```python
from build123d import *

# Parameters (mm, degrees)
PAD008_DEPTH    = 50
SKETCH046_R     = 2.4
SKETCH046_R_2   = 2
POCKET024_DEPTH = 30
SKETCH047_W     = 30
SKETCH047_H     = 35
POCKET025_DEPTH = 30
POCKET026_DEPTH = 5
FILLET014_R     = 4
FILLET015_R     = 1
FILLET016_R     = 1


with BuildPart() as part:
    # Sketch045 → Pad008 (new body)
    with BuildSketch(Plane.XZ):
        with BuildLine():
            Line((0, 47), (0, -18))
            ThreePointArc((0, -18), (0.585786, -19.414214), (2, -20))
            Line((2, -20), (23, -20))
            Line((23, -20), (23, -17.9))
            Line((17, -17.9), (23, -17.9))
            Line((17, -4.9), (17, -17.9))
            Line((17, -4.9), (23, -4.9))
            Line((23, -4.9), (23, -2))
            Line((23, -2), (9, -2))
            ThreePointArc((4, 3), (5.464466, -0.535534), (9, -2))
            Line((4, 3), (4, 47))
            Line((4, 47), (0, 47))
        make_face()
    extrude(amount=-PAD008_DEPTH)

    # Sketch046 → Pocket024 (cut)
    with BuildSketch(Plane.YZ):
        with Locations((10, -11.4)):
            Circle(SKETCH046_R)
        with Locations((10, 25)):
            Circle(SKETCH046_R_2)
        with Locations((40, 25)):
            Circle(SKETCH046_R_2)
    extrude(amount=POCKET024_DEPTH, mode=Mode.SUBTRACT)

    # Sketch047 → Pocket025 (cut)
    with BuildSketch(Plane.YZ.offset(4)):
        with Locations((35, -2.5)):
            Rectangle(SKETCH047_W, SKETCH047_H)
    extrude(amount=POCKET025_DEPTH, mode=Mode.SUBTRACT)

    # Sketch048 → Pocket026 (cut)
    with BuildSketch(Plane.YZ):
        Polygon((5.438933, -11.4), (7.719466, -15.35), (12.280534, -15.35), (14.561067, -11.4), (12.280534, -7.45), (7.719466, -7.45), align=None)
    extrude(amount=POCKET026_DEPTH, mode=Mode.SUBTRACT)

    # Fillet014
    fillet014_edges = [part.edges().sort_by_distance(p)[0] for p in [
        (4, 20, -8.5),
    ]]
    fillet(fillet014_edges, radius=FILLET014_R)

    # Fillet015
    fillet015_edges = [part.edges().sort_by_distance(p)[0] for p in [
        (20, 0, -4.9),
        (23, 10, -4.9),
        (17, 10, -4.9),
        (20, 20, -4.9),
        (17, 20, -11.4),
        (17, 0, -11.4),
        (23, 10, -17.9),
        (17, 10, -17.9),
        (20, 20, -17.9),
        (20, 0, -17.9),
    ]]
    fillet(fillet015_edges, radius=FILLET015_R)

    # Fillet016
    fillet016_edges = [part.edges().sort_by_distance(p)[0] for p in [
        (0, 0, 14.5),
        (0, 25, 47),
        (0, 50, 14.5),
    ]]
    fillet(fillet016_edges, radius=FILLET016_R)


solid = part.part
```
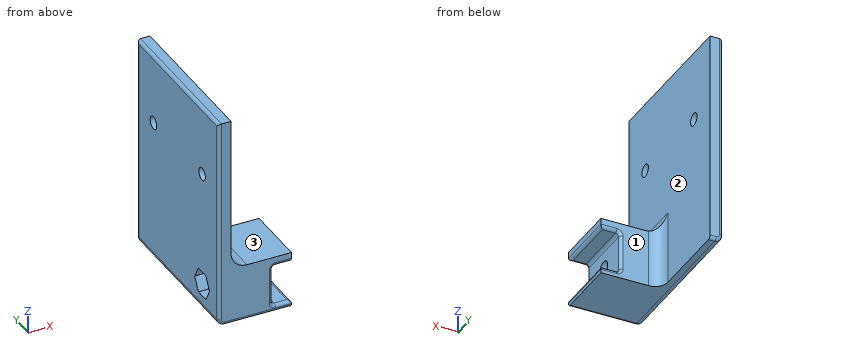
Verification items for the finished model (mm, model axes). Face numbers are marked on the shaded views. A direction names the side the tool comes from. Round coordinates to 2 decimals unless told otherwise and drop trailing zeros. Order: outer loops, then holes, each group sorted by start corner. A loop starts at its lowest first (then second) coordinate and runs counter-clockwise, first axis right, second up.
1) Depth check by flat-ended pin: pin 1 (4.5 mm diameter, centred on x = 16.5, z = -8.5, fed in from +Y); pin 2 (4.5 mm diameter, centred on x = 19.5, y = 9, fed in from +Z); pin 3 (4.5 mm diameter, centred on y = 10, z = -11.4, fed in from +X); pin 4 (1.5 mm diameter, centred on y = 9.5, z = 20, fed in from +X). Enter the tip coordinate at first touch or a pass-through.
Geometry says:
pin 1: stops at y = 20
pin 2: stops at z = -2
pin 3: passes through
pin 4: stops at x = 4
2) Material ranges on line 1 (Y direction, x = 1.4, z = 25); line 2 (Z direction, x = 18.75, y = 12.5); line 3 (Z direction, x = 1.85, y = 40), recorded low to high.
Geometry says:
line 1: y = 0 to 8, 12 to 38, 42 to 50
line 2: z = -20 to -17.9, -4.9 to -2
line 3: z = -19.99 to 23, 27 to 47
3) Cross-section at B-B, the plane z = 25. Record the cut outline in (x, y).
Geometry says:
outline: (0, 1) arc R1 ccw to (1, 0) - (4, 0) - (4, 8) - (0, 8) - close; (0, 12) - (4, 12) - (4, 38) - (0, 38) - close; (0, 42) - (4, 42) - (4, 50) - (1, 50) arc R1 ccw to (0, 49) - close
4) Tool access check on the marked faces 1, 2 and 3. Record the directions out of +Z, -Z, +X, -X, +Y, -Y that give a thin tool (end or side, any length) a straight path to the whole face; none if there is none.
Geometry says:
face 1: +Z, -Z, +X, +Y
face 2: +Z, +X, +Y
face 3: +Z, +X, +Y, -Y
5) Cross-section at D-D, the plane x = 21. Record the cut outline in (y, z).
Geometry says:
outline: (0, -19) arc R1 ccw to (1, -20) - (20, -20) - (20, -18.9) arc R1 ccw to (19, -17.9) - (1, -17.9) arc R1 ccw to (0, -18.9) - close; (0, -3.9) arc R1 ccw to (1, -4.9) - (19, -4.9) arc R1 ccw to (20, -3.9) - (20, -2) - (0, -2) - close
6) Cross-section at C-C, the plane y = 10. Give the number of separate pieces and of enclosed holes in the cut face, plus the area to 3 significant figures.
Geometry says:
separate pieces: 3
enclosed holes: 0
area: 423 mm2
7) Cross-section at A-A, the plane y = 40. Record the cut outline in (x, z), plus the area to 3 significant figures.
Geometry says:
outline: (0, -18) arc R2 ccw to (2, -20) - (4, -20) - (4, 23) - (0, 23) - close; (0, 27) - (4, 27) - (4, 47) - (1, 47) arc R1 ccw to (0, 46) - close
area: 251 mm2
